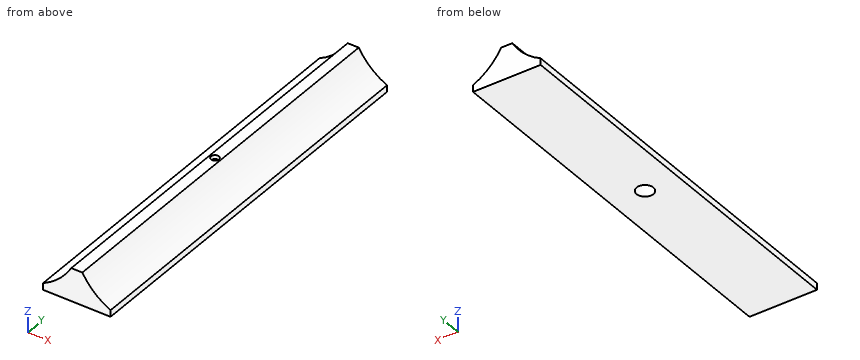
from build123d import *

# Parameters (mm, degrees)
BOSS_EXTRUDE1_DEPTH                       = 30
TAPPED_HOLE_FOR_M2_5X0_45_HELICOIL1_D     = 2.55
TAPPED_HOLE_FOR_M2_5X0_45_HELICOIL1_DEPTH = 4
TAPPED_HOLE_FOR_M2_5X0_45_HELICOIL1_TIP   = 0.766097289
F_1_2_1_2_DIAMETER_HOLE1_D                = 1.2
F_1_2_1_2_DIAMETER_HOLE1_DEPTH            = 6.45
F_1_2_1_2_DIAMETER_HOLE1_TIP              = 0.360516371


with BuildPart() as part:
    # Sketch1 → Boss-Extrude1 (new, symmetric)
    with BuildSketch(Plane(origin=(0, 0, 0), x_dir=(1, 0, 0), z_dir=(0, 1, 0))):
        with BuildLine():
            Line((-0.839745962, 0), (0.839745962, 0))
            ThreePointArc((0.839745962, 0), (2.690111154, 2.322937519), (5.141101056, 4))
            Line((5.141101056, 4), (5.141101056, 5))
            Line((5.141101056, 5), (-5.141101056, 5))
            Line((-5.141101056, 5), (-5.141101056, 4))
            ThreePointArc((-5.141101056, 4), (-2.690111154, 2.322937519), (-0.839745962, 0))
        make_face()
    extrude(amount=BOSS_EXTRUDE1_DEPTH, both=True)

    # Tapped Hole for M2.5x0.45 Helicoil1
    with Locations(Plane(origin=(0, 0, -5), x_dir=(-1, 0, 0), z_dir=(0, 0, -1))):
        with Locations((0, 0)):
            Hole(TAPPED_HOLE_FOR_M2_5X0_45_HELICOIL1_D / 2, depth=TAPPED_HOLE_FOR_M2_5X0_45_HELICOIL1_DEPTH)
            with Locations((0, 0, -(TAPPED_HOLE_FOR_M2_5X0_45_HELICOIL1_DEPTH + TAPPED_HOLE_FOR_M2_5X0_45_HELICOIL1_TIP / 2))):  # 118° drill point
                Cone(0, TAPPED_HOLE_FOR_M2_5X0_45_HELICOIL1_D / 2, TAPPED_HOLE_FOR_M2_5X0_45_HELICOIL1_TIP, mode=Mode.SUBTRACT)

    # Ø1.2 (1.2) Diameter Hole1
    with Locations(Plane(origin=(0, 0, -5), x_dir=(-1, 0, 0), z_dir=(0, 0, -1))):
        with Locations((0, 0)):
            Hole(F_1_2_1_2_DIAMETER_HOLE1_D / 2, depth=F_1_2_1_2_DIAMETER_HOLE1_DEPTH)
            with Locations((0, 0, -(F_1_2_1_2_DIAMETER_HOLE1_DEPTH + F_1_2_1_2_DIAMETER_HOLE1_TIP / 2))):  # 118° drill point
                Cone(0, F_1_2_1_2_DIAMETER_HOLE1_D / 2, F_1_2_1_2_DIAMETER_HOLE1_TIP, mode=Mode.SUBTRACT)


solid = part.part
Work out the finished part from the listing and answer in its coordinate system (mm). Give positions to 0.01 mm unless a question says otherwise; leave off trailing zeros. Loops run counter-clockwise (first coordinate to the right, second up) from the corner with the lowest first, then second, coordinate; pieces in that order, holes last. Notation, with made-up numbers: (76, 84.5) -> (102, 84.5) arc R14 cw to (102, 89.5) -> close; hole circle Ø1 at (39.25, -33). An arc over 180 degrees is marked (long way). Use a Markdown table: item, result. Add a question column.
1. Find the intervals of material crossed by probe 1 along X at (y, z) = (0, -4.05) (3 decimals); probe 2 along Y at (x, z) = (0, -0.4); probe 3 along X at (y, z) = (0, -2.35) (3 decimals), in increasing order.
2. Flat-ended cylindrical pins translate along their axes: pin 1 Ø3 at (x, y) = (4, -20.5) entering from +Z; pin 2 Ø1.9 at (x, y) = (0, 0) entering from -Z. Find the tip coordinate at first contact, or state that the pin passes through.
3. Section A-A on y = 0 is taken. Determine the outline of the cut face in (x, z) (3 decimals), and give its area (3 significant figures).
4. Section B-B on x = 0 is taken. Determine the outline of the cut face in (y, z) (3 decimals).
5. Section D-D on y = -18 is taken. Determine the outline of the cut face in (x, z).
6. Section C-C on z = -1.75 is taken. Determine the outline of the cut face in (x, y) (3 decimals).
Results below:
| question | item | result |
|---|---|---|
| 1 | probe 1 | x = -5.141 to -1.275, 1.275 to 5.141 |
| 1 | probe 2 | y = -30 to -0.6, 0.6 to 30 |
| 1 | probe 3 | x = -2.719 to -1.275, 1.275 to 2.719 |
| 2 | pin 1 | stops at z = -2.14 |
| 2 | pin 2 | stops at z = -0.8 |
| 3 | outline | (-5.141, -5) -> (-1.275, -5) -> (-1.275, -1) -> (-0.6, -0.594) -> (-0.6, 0) -> (-0.84, 0) arc R10 cw to (-5.141, -4) -> close; (0.6, -0.594) -> (1.275, -1) -> (1.275, -5) -> (5.141, -5) -> (5.141, -4) arc R10 cw to (0.84, 0) -> (0.6, 0) -> close |
| 3 | area | 19.1 mm^2 |
| 4 | outline | (-30, -5) -> (-1.275, -5) -> (-1.275, -1) -> (-0.6, -0.594) -> (-0.6, 0) -> (-30, 0) -> close; (0.6, -0.594) -> (1.275, -1) -> (1.275, -5) -> (30, -5) -> (30, 0) -> (0.6, 0) -> close |
| 5 | outline | (-5.14, -5) -> (5.14, -5) -> (5.14, -4) arc R10 cw to (0.84, 0) -> (-0.84, 0) arc R10 cw to (-5.14, -4) -> close |
| 6 | outline | (-2.122, -30) -> (2.122, -30) -> (2.122, 30) -> (-2.122, 30) -> close; hole circle Ø2.55 at (0, 0) |
